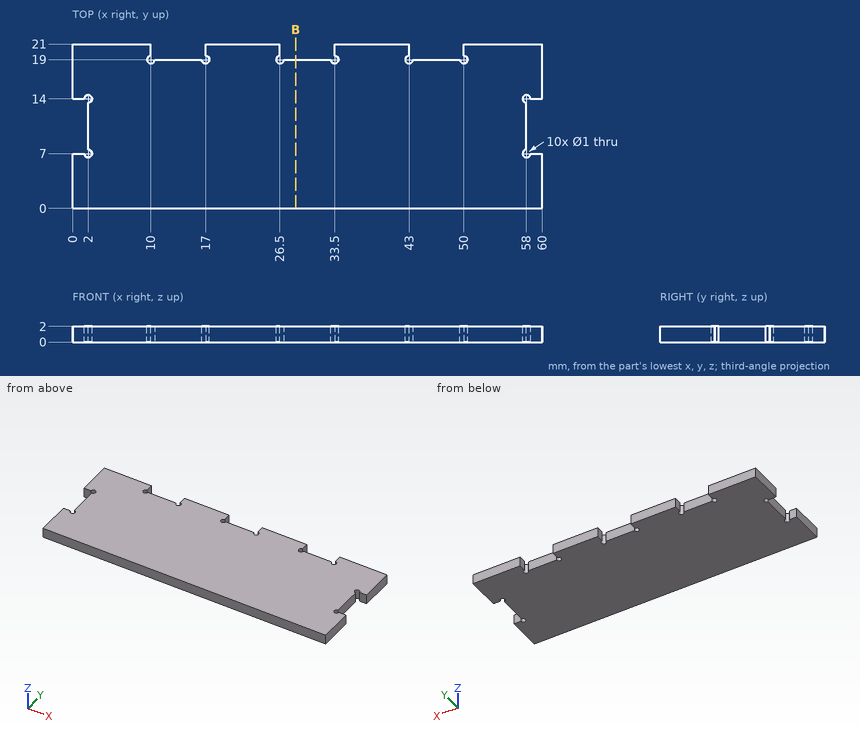
Design review of the part shown in the three views and the two pictorial views. Dimensions are in mm from the part's minimum x, y and z. Coordinates: 2 decimals unless noted, no trailing zeros. Order: outer loops, then holes, each group sorted by start corner. A loop starts at its lowest first (then second) coordinate and runs counter-clockwise, first axis right, second up.
Item 1: For line 1 (X direction, y = 9, z = 0.15); line 2 (Y direction, x = 48, z = 1.3), list the stretches that pass through material, from the lowest coordinate up.
Item 2: Take a section at B-B, the plane x = 28.5. Write out the cut boundary in (y, z), then the cut area to 3 significant figures.
Item 3: For pin 1 Ø1.2 at (y, z) = (20.5, 1.5) entering from -X; pin 2 Ø0.6 at (x, z) = (29, 1) entering from +Y; pin 3 Ø0.6 at (y, z) = (9.5, 1) entering from -X, all flat-tipped, find the tip position at first contact; note any pin that passes through.
The answers:
1. line 1: x = 2 to 58
1. line 2: y = 0 to 19
2. outline: (0, 0) - (19, 0) - (19, 2) - (0, 2) - close
2. area: 38.0 mm2
3. pin 1: stops at x = 0
3. pin 2: stops at y = 19
3. pin 3: stops at x = 2
